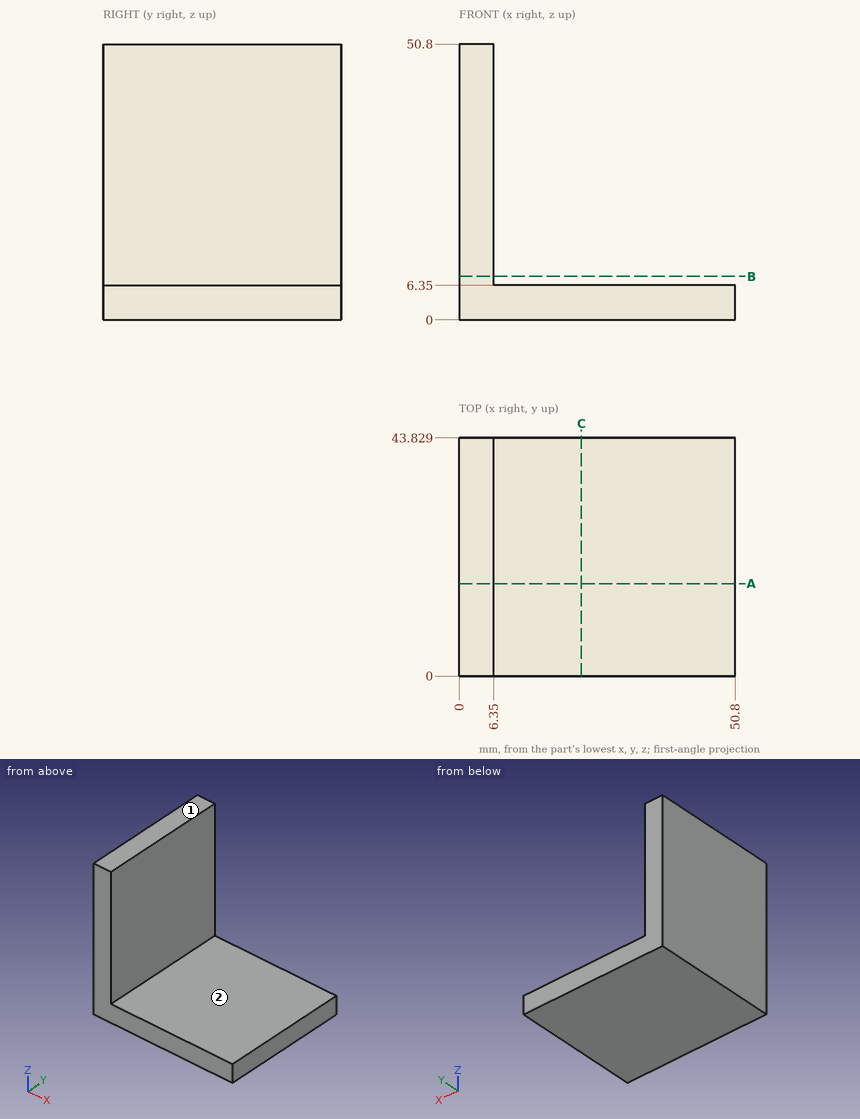
Input: dimensioned drawing with shaded views. Units: mm. Origin: part minimum x, y, z. A direction names the side the tool comes from. Give positions to 0.01 mm unless a question says otherwise; leave off trailing zeros. Write each loop counter-clockwise with the first axis right and the second up, starting at its lowest first coordinate (ties: lowest second). Pieces come first, ordered by that corner, then holes.
Q1. Set-up query: the marked faces 1 and 2. Return all of +Z, -Z, +X, -X, +Y, -Y with unobstructed straight access to the full face (end or side cutting, diameter ignored); none if empty.
Q2. First-contact query: P1, Ø8, axis at x = 33.5, y = 14, coming from the -Z side; P2, Ø6, axis at y = 29.5, z = 10, coming from the +X side. Flat tips, straight axial feed; report the tip coordinate or a pass-through.
Q3. Section C-C, the plane x = 22.5. Output: boundary loops of the cut face in (y, z).
Q4. Section A-A, the plane y = 17. Output: boundary loops of the cut face in (x, z).
Q5. Material intervals for probe 1 along Z at (x, y) = (21.5, 35), sorted ascending.
Q6. Section B-B, the plane z = 8. Output: boundary loops of the cut face in (x, y), plus the area to 3 significant figures.
Filled in:
1. face 1: +Z, +X, -X, +Y, -Y
1. face 2: +Z, +X, +Y, -Y
2. P1: stops at z = 0
2. P2: stops at x = 6.35
3. outline: (0, 0) - (43.83, 0) - (43.83, 6.35) - (0, 6.35) - close
4. outline: (0, 0) - (50.8, 0) - (50.8, 6.35) - (6.35, 6.35) - (6.35, 50.8) - (0, 50.8) - close
5. probe 1: z = 0 to 6.35
6. outline: (0, 0) - (6.35, 0) - (6.35, 43.83) - (0, 43.83) - close
6. area: 278 mm2
